```python
from build123d import *

# Parameters (mm, degrees)
ESQUISSE1_W             = 30
ESQUISSE1_H             = 19.2
ESQUISSE1_W_2           = 25.6
ESQUISSE1_H_2           = 14.8
BOSS_EXTRU_1_DEPTH      = 63.5
BOSS_EXTRU_1_DEPTH_BACK = 63.5
CONG_3_R                = 4


with BuildPart() as part:
    # Esquisse1 → Boss.-Extru.1 (new body, two sides)
    with BuildSketch(Plane.XY) as boss_extru_1_sk:
        Rectangle(ESQUISSE1_W, ESQUISSE1_H)
        Rectangle(ESQUISSE1_W_2, ESQUISSE1_H_2, mode=Mode.SUBTRACT)
    extrude(amount=BOSS_EXTRU_1_DEPTH)
    extrude(boss_extru_1_sk.sketch, amount=-BOSS_EXTRU_1_DEPTH_BACK)

    # Cong_3
    cong_3_edges = [part.edges().sort_by_distance(p)[0] for p in [
        (12.8, 7.4, 0),
        (12.8, -7.4, 0),
        (-12.8, -7.4, 0),
        (-12.8, 7.4, 0),
        (15, -9.6, 0),
        (-15, -9.6, 0),
        (-15, 9.6, 0),
        (15, 9.6, 0),
    ]]
    fillet(cong_3_edges, radius=CONG_3_R)


solid = part.part
```
Design review of the part built by this model. Coordinates are the model's own, in mm. A direction names the side the tool comes from. Coordinates: 2 decimals unless noted, no trailing zeros. Order: outer loops, then holes, each group sorted by start corner. A loop starts at its lowest first (then second) coordinate and runs counter-clockwise, first axis right, second up. Notation, with made-up numbers: (87.5, 81) - (112.5, 81) arc R15 cw to (112.5, 86) - close; hole circle Ø8 at (43, 61). An arc over 180 degrees is marked (long way). Answer in a Markdown table with one row per item.
(1) Wall thickness on line 1 along X through (y, z) = (-3.5, -47); line 2 along Y through (x, z) = (8, -20); line 3 along Y through (x, z) = (-10.5, 5): over which ranges is each line inside the solid? List them lowest first. Write a range as from..to.
Checked values:
| item | result |
|---|---|
| line 1 | -15..-12.8, 12.8..15 |
| line 2 | -9.6..-7.4, 7.4..9.6 |
| line 3 | -9.6..-7.02, 7.02..9.6 |
(2) Consider section A-A on z = 23.5. State the section outline as (x, y) points.
Checked values:
| item | result |
|---|---|
| outline | (-15, -5.6) arc R4 ccw to (-11, -9.6) - (11, -9.6) arc R4 ccw to (15, -5.6) - (15, 5.6) arc R4 ccw to (11, 9.6) - (-11, 9.6) arc R4 ccw to (-15, 5.6) - close; hole (-12.8, -3.4) arc R4 ccw to (-8.8, -7.4) - (8.8, -7.4) arc R4 ccw to (12.8, -3.4) - (12.8, 3.4) arc R4 ccw to (8.8, 7.4) - (-8.8, 7.4) arc R4 ccw to (-12.8, 3.4) - close |
(3) Consider section B-B on x = 1.25. State the section outline as (y, z) points, plus the area to 3 significant figures.
Checked values:
| item | result |
|---|---|
| outline | (-9.6, -63.5) - (-7.4, -63.5) - (-7.4, 63.5) - (-9.6, 63.5) - close; (7.4, -63.5) - (9.6, -63.5) - (9.6, 63.5) - (7.4, 63.5) - close |
| area | 559 mm^2 |
(4) For faces 1 (the flat face through (0, -7.4, 1)), 2 (the flat face through (0, -8, -63.5)), list the 3-axis set-ups (+Z, -Z, +X, -X, +Y, -Y) from which the entire face can be reached by the end or side of a thin tool; tool diameter is ignored.
Checked values:
| item | result |
|---|---|
| face 1 | +Z, -Z |
| face 2 | -Z, +X, -X, +Y, -Y |
(5) The part is to be moulded in two halves that separate along Y. For faces 3 (the flat face through (-15, 0, 1)), 4 (the flat face through (0, 9.6, 1)), 5 (the flat face through (0, 7.4, 1)), 6 (the flat face through (12.8, 0, 1)), say which applies: released by +Y, released by -Y, zero draft, split by the parting line, or undercut.
Checked values:
| item | result |
|---|---|
| face 3 | zero draft |
| face 4 | released by +Y |
| face 5 | undercut |
| face 6 | undercut |
